```python
from build123d import *

# Parameters (mm, degrees)
F0_W     = 24
F0_H     = 4
F0_R     = 2
F1_DEPTH = 2.5
F2_W     = 20
F2_H     = 3
F3_DEPTH = 25
F4_SIZE  = 2.49999


# Not quite as in the source:
# - a fillet or chamfer is up to 0.001 mm smaller than in the source, because OpenCascade refuses the exact size


with BuildPart() as f1:
    # F0 (on Top) → F1 (new body)
    with BuildSketch(Plane.XY):
        with BuildLine():
            Line((-36.8828806926, 6.1976464093), (-51.8828806926, 6.1976464093))
            ThreePointArc((-51.8828806926, 6.1976464093), (-55.4184145986, 4.7331803152), (-56.8828806926, 1.1976464093))
            Line((-56.8828806926, 1.1976464093), (-56.8828806926, -26.8023535907))
            ThreePointArc((-56.8828806926, -26.8023535907), (-55.4184145986, -30.3378874967), (-51.8828806926, -31.8023535907))
            Line((-51.8828806926, -31.8023535907), (-8.8828806926, -31.8023535907))
            Line((-8.8828806926, -31.8023535907), (-8.8828806926, -27.8023535907))
            Line((-8.8828806926, -27.8023535907), (15.1171193074, -27.8023535907))
            Line((15.1171193074, -27.8023535907), (15.1171193074, -31.8023535907))
            Line((15.1171193074, -31.8023535907), (58.1171193074, -31.8023535907))
            ThreePointArc((58.1171193074, -31.8023535907), (61.6526532133, -30.3378874967), (63.1171193074, -26.8023535907))
            Line((63.1171193074, -26.8023535907), (63.1171193074, 1.1976464093))
            ThreePointArc((63.1171193074, 1.1976464093), (61.6526532133, 4.7331803152), (58.1171193074, 6.1976464093))
            Line((58.1171193074, 6.1976464093), (43.1171193074, 6.1976464093))
            Line((43.1171193074, 6.1976464093), (23.1171193074, 6.1976464093))
            Line((23.1171193074, 6.1976464093), (23.1171193074, 41.1976464093))
            ThreePointArc((23.1171193074, 41.1976464093), (21.6526532133, 44.7331803152), (18.1171193074, 46.1976464093))
            Line((18.1171193074, 46.1976464093), (10.6171193074, 46.1976464093))
            Line((10.6171193074, 46.1976464093), (10.6171193074, 42.1976464093))
            Line((10.6171193074, 42.1976464093), (-4.3828806926, 42.1976464093))
            Line((-4.3828806926, 42.1976464093), (-4.3828806926, 46.1976464093))
            Line((-4.3828806926, 46.1976464093), (-11.8828806926, 46.1976464093))
            ThreePointArc((-11.8828806926, 46.1976464093), (-15.4184145986, 44.7331803152), (-16.8828806926, 41.1976464093))
            Line((-16.8828806926, 41.1976464093), (-16.8828806926, 6.1976464093))
            Line((-16.8828806926, 6.1976464093), (-36.8828806926, 6.1976464093))
        make_face()
        with Locations((3.1171193074, 4.1976464093)):
            Rectangle(F0_W, F0_H, mode=Mode.SUBTRACT)
        with Locations((-11.8828806926, 11.1976464093)):
            Circle(F0_R, mode=Mode.SUBTRACT)
        with Locations((-11.8828806926, 41.1976464093)):
            Circle(F0_R, mode=Mode.SUBTRACT)
        with Locations((18.1171193074, 11.1976464093)):
            Circle(F0_R, mode=Mode.SUBTRACT)
        with Locations((18.1171193074, 41.1976464093)):
            Circle(F0_R, mode=Mode.SUBTRACT)
        with BuildLine():
            Line((-36.8828806926, 41.1976464093), (-36.8828806926, 6.1976464093))
            Line((-36.8828806926, 6.1976464093), (-16.8828806926, 6.1976464093))
            Line((-16.8828806926, 6.1976464093), (-16.8828806926, 41.1976464093))
            ThreePointArc((-16.8828806926, 41.1976464093), (-15.4184145986, 44.7331803152), (-11.8828806926, 46.1976464093))
            Line((-11.8828806926, 46.1976464093), (-16.8828806926, 46.1976464093))
            Line((-16.8828806926, 46.1976464093), (-31.8828806926, 46.1976464093))
            ThreePointArc((-31.8828806926, 46.1976464093), (-35.4184145986, 44.7331803152), (-36.8828806926, 41.1976464093))
        make_face()
        with BuildLine():
            Line((23.1171193074, 46.1976464093), (18.1171193074, 46.1976464093))
            ThreePointArc((18.1171193074, 46.1976464093), (21.6526532133, 44.7331803152), (23.1171193074, 41.1976464093))
            Line((23.1171193074, 41.1976464093), (23.1171193074, 6.1976464093))
            Line((23.1171193074, 6.1976464093), (43.1171193074, 6.1976464093))
            Line((43.1171193074, 6.1976464093), (43.1171193074, 41.1976464093))
            ThreePointArc((43.1171193074, 41.1976464093), (41.6526532133, 44.7331803152), (38.1171193074, 46.1976464093))
            Line((38.1171193074, 46.1976464093), (23.1171193074, 46.1976464093))
        make_face()
    extrude(amount=F1_DEPTH)

    # F2 (on face) → F3 (cut)
    with BuildSketch(Plane.XY.offset(2.5)):
        with Locations((-26.8828806926, 7.6976464093)):
            Rectangle(F2_W, F2_H)
        with Locations((33.1171193074, 7.6976464093)):
            Rectangle(F2_W, F2_H)
    extrude(amount=-F3_DEPTH, mode=Mode.SUBTRACT)

    # F4 (size 2.5 in the source; OpenCascade refuses exactly that, so slightly less here)
    f4_edges = [f1.edges().sort_by_distance(p)[0] for p in [
        (3.117119, 42.197646, 2.5),
    ]]
    chamfer(f4_edges, length=F4_SIZE)


solid = f1.part
```
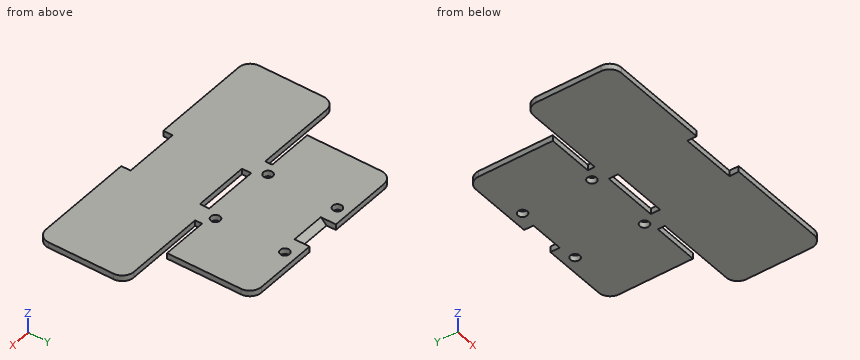
Verification items for the finished model (mm, model axes). Give positions to 0.01 mm unless a question says otherwise; leave off trailing zeros. Write each loop counter-clockwise with the first axis right and the second up, starting at its lowest first coordinate (ties: lowest second). Pieces come first, ordered by that corner, then holes. Notation, with made-up numbers: M -36.75,75 L 22.25,75 A7 ccw 22.25,82 Z; hole C 4,61.5 d10. An arc over 180 degrees is marked long. One line per question, with ' | ' between items.
1) Thickness scan on line 1 along Y through (x, z) = (16.5, 0.7); line 2 along Y through (x, z) = (-25.5, 1.5); line 3 along X through (y, z) = (29.5, 1.75). Record the ranges inside material, lowest first. Write a range as [from, to].
Result:
line 1: y = [-31.8, 10.02], [12.37, 40.02], [42.37, 46.2] | line 2: y = [-31.8, 6.2], [9.2, 46.2] | line 3: x = [-36.88, 43.12]
2) Section check D-D on y = 18. Enter the section's corners in (x, z).
Result:
outline: M -36.88,0 L 43.12,0 L 43.12,2.5 L -36.88,2.5 Z
3) Section check A-A on x = -24. Enter the section's corners in (y, z).
Result:
outline: M -31.8,0 L 6.2,0 L 6.2,2.5 L -31.8,2.5 Z; M 9.2,0 L 46.2,0 L 46.2,2.5 L 9.2,2.5 Z
4) Gauge pin test, flat ends, axial feed: pin 1 Ø0.8 at (x, z) = (6, 1.5) entering from -Y; pin 2 Ø1.2 at (y, z) = (7.5, 2) entering from -X; pin 3 Ø1.2 at (y, z) = (4.5, 1.5) entering from +X; pin 4 Ø3.5 at (x, y) = (-11.88, 11.2) entering from -Z. Record the tip position at first contact, or that the pin passes through.
Result:
pin 1: stops at y = -27.8 | pin 2: stops at x = -16.88 | pin 3: stops at x = 62.32 | pin 4: passes through
5) Section check B-B on z = 1.6. State how many separate pieces and enclosed holes the cut face has, plus the area to 3 significant figures.
Result:
separate pieces: 1 | enclosed holes: 5 | area: 7,280 mm2
